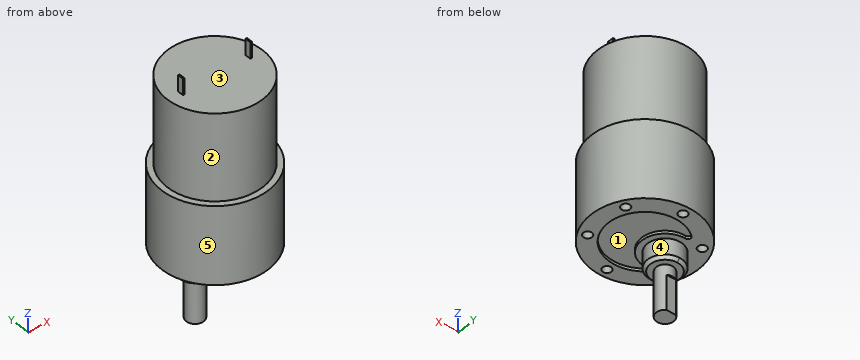
Autodesk Inventor part; units mm, degrees
ref_plane "YZ Plane" through (0, 0, 0) normal (1, 0, 0) x (0, 1, 0)
ref_plane "XZ Plane" through (0, 0, 0) normal (0, 1, 0) x (-1, 0, 0)
ref_plane "XY Plane" through (0, 0, 0) normal (0, 0, 1) x (1, 0, 0)
sketch "Boceto1" plane through (0, 0, 0) normal (0, 0, 1) x (1, 0, 0)
  circle A0 centre (0, 0) radius 18.4
  dimension "d0" = 36.8
extrude "Extrusión1" add sketch "Boceto1" along normal blind 27
sketch "Boceto2" plane through (0, 0, 27) normal (0, 0, 1) x (1, 0, 0)
  circle A0 centre (0, 0) radius 18.4
  circle A1 centre (0, 0) radius 16.4
  dimension "d4" = 2
extrude "Extrusión2" add sketch "Boceto2" along normal blind 30 contours A1
sketch "Boceto3" plane through (0, 0, 57) normal (0, 0, 1) x (1, 0, 0)
  circle A0 centre (0, 0) radius 16.4
  line L0 (0, 0) -> (12.05, 0)
  line L1 (0, 0) -> (-12.05, 0)
  line L2 (-12.05, 0) -> (-12.05, 1)
  line L3 (-12.05, 1) -> (-12, 1)
  line L4 (-12, 1) -> (-12, -1)
  line L5 (-12, -1) -> (-12.05, -1)
  line L6 (-12.05, -1) -> (-12.05, 0)
  line L7 (12.05, 0) -> (12.05, 1)
  line L8 (12.05, 1) -> (12, 1)
  line L9 (12, 1) -> (12, -1)
  line L10 (12, -1) -> (12.05, -1)
  line L11 (12.05, -1) -> (12.05, 0)
  dimension "d7" = 12.05
  dimension "d8" = 12.05
extrude "Extrusión3" add sketch "Boceto3" along normal blind 5.6 contours L9 L8 L7 L0 | L0 L11 L10 L9 | L4 L5 L6 L1 | L1 L2 L3 L4
sketch "Boceto4" plane through (0, 0, 0) normal (0, 0, -1) x (-1, 0, 0)
  circle A0 centre (13.4234, -7.75) radius 1.5
  circle A1 centre (13.4234, 7.75) radius 1.5
  circle A2 centre (0, 15.5) radius 1.5
  circle A3 centre (-13.4234, 7.75) radius 1.5
  circle A4 centre (-13.4234, -7.75) radius 1.5
  circle A5 centre (0, -15.5) radius 1.5
  line L0 (0, 0) -> (7, 0)
  circle A6 centre (7, 0) radius 6
  arc A7 (7.2895, 7.9948) -> (7.2895, -7.9948) centre (7, 0) ccw
  arc A8 (7.9572, 9.7695) -> (7.9572, -9.7695) centre (0, 0) ccw
  arc A9 (7.9572, -9.7695) -> (7.2895, -7.9948) centre (7.3257, -8.9941) ccw
  arc A10 (7.2895, 7.9948) -> (7.9572, 9.7695) centre (7.3257, 8.9941) ccw
  dimension "d19" = 7
  dimension "d20" = 12
  dimension "d34" = 1
extrude "Extrusión4" add sketch "Boceto4" along normal blind 6 contours A6
sketch "Boceto5" plane through (-7, 0, -6) normal (0, 0, -1) x (-1, 0, 0)
  circle A0 centre (0, 0) radius 6
  line L0 (6, 0) -> (0, 0)
  line L1 (0, 6) -> (0, 0)
extrude "Extrusión5" add sketch "Boceto5" along normal blind 0.5 contours L0 L1 A0 picked at (3.9499, 0.445)
sketch "Boceto6" plane through (0, 0, -6) normal (0, 0, -1) x (-1, 0, 0)
  line L0 (13, 0) -> (7, 0)
  line L1 (7, 0) -> (7, 6)
  arc A0 (7, 6) -> (13, 0) centre (7, 0) ccw
extrude "Extrusión6" cut sketch "Boceto6" against normal blind 0.5
sketch "Boceto7" plane through (-7, 0, -6.5) normal (1, 0, 0) x (0, 0, -1)
  line L0 (0, 0) -> (0, 6)
  line L1 (-1, 0) -> (0, 0)
  line L2 (-1, 6) -> (0, 5)
  line L3 (0, 5) -> (0, 6)
  line L4 (-1, 6) -> (0, 5)
  line L5 (-1, 6) -> (0, 6)
  line L6 (-1, 6) -> (0, 5)
  line L7 (0, 5) -> (-1, 6)
revolve "Revolución1" cut sketch "Boceto7" angle 360 about axis through (-7, 0, -5.5) along (0, 0, -1)
sketch "Boceto8" plane through (-7, 0, -5.5) normal (1, 0, 0) x (0, 0, -1)
  line L0 (1, 5) -> (0, 6)
  line L1 (0, 0) -> (0, 6)
  line L2 (0, 0) -> (1, 0)
  line L3 (1, 0) -> (1, 5)
revolve "Revolución2" add sketch "Boceto8" angle 360 about axis through (-7, 0, -5.5) along (0, 0, -1)
sketch "Boceto9" plane through (-7, 0, -6.5) normal (0, 0, -1) x (-1, 0, 0)
  circle A0 centre (0, 0) radius 5
  circle A1 centre (0, 0) radius 3
extrude "Extrusión7" add sketch "Boceto9" along normal blind 15.5 contours A1
sketch "Boceto10" plane through (-7, 0, -22) normal (0, 0, -1) x (-1, 0, 0)
  circle A0 centre (0, 0) radius 3
  line L0 (1.6583, 2.5) -> (-1.6583, 2.5)
extrude "Extrusión8" cut sketch "Boceto10" against normal blind 12 contours L0 A0 picked at (-0.1169, 2.6598)
extrude "Extrusión9" cut sketch "Boceto4" against normal blind 1 contours A7 A9 A8 A10
extrude "Extrusión10" cut sketch "Boceto4" against normal blind 10 contours A0 | A1 | A2 | A3 | A4 | A5
sketch "Boceto12" plane through (-12, -1, 57) normal (1, 0, 0) x (0, 0, -1)
  line L0 (-5.6, 2) -> (-5.6, 0)
  line L1 (0, 0) -> (-5.6, 0)
  line L2 (0, 2) -> (0, 0)
  line L3 (0, 2) -> (-5.6, 2)
extrude "Extrusión11" add sketch "Boceto12" along normal blind 0.45
sketch "Boceto13" plane through (12, -1, 57) normal (-1, 0, 0) x (0, 0, 1)
  line L0 (5.6, 0) -> (5.6, 2)
  line L1 (0, 2) -> (5.6, 2)
  line L2 (0, 0) -> (0, 2)
  line L3 (0, 0) -> (5.6, 0)
extrude "Extrusión12" add sketch "Boceto13" along normal blind 0.45
sketch "Boceto14" plane through (0, 0, 0) normal (0, 0, -1) x (-1, 0, 0)
  circle A0 centre (0, -15.5) radius 1.5
  circle A1 centre (-13.4234, -7.75) radius 1.5
  circle A2 centre (-13.4234, 7.75) radius 1.5
  circle A3 centre (13.4234, 7.75) radius 1.5
  circle A4 centre (13.4234, -7.75) radius 1.5
  circle A5 centre (0, 15.5) radius 1.5
  arc A6 (7.2895, 7.9948) -> (7.2895, -7.9948) centre (7, 0) ccw
  arc A7 (7.9572, -9.7695) -> (7.2895, -7.9948) centre (7.3257, -8.9941) ccw
  arc A8 (7.9572, 9.7695) -> (7.9572, -9.7695) centre (0, 0) ccw
  arc A9 (7.2895, 7.9948) -> (7.9572, 9.7695) centre (7.3257, 8.9941) ccw
  circle A10 centre (7, 0) radius 6
  circle A11 centre (0, 0) radius 18.4
sketch "Boceto15" plane through (-7, 0, -22) normal (0, 0, -1) x (-1, 0, 0)
  line L0 (1.6583, 2.5) -> (-1.6583, 2.5)
  arc A0 (-1.6583, 2.5) -> (1.6583, 2.5) centre (0, 0) ccw
properties part number "37D"
Work out the finished part from the listing and answer in its coordinate system (mm). Face numbers are marked on the shaded views. A direction names the side the tool comes from. Round coordinates to 2 decimals unless told otherwise and drop trailing zeros. Loops run counter-clockwise (first coordinate to the right, second up) from the corner with the lowest first, then second, coordinate; pieces in that order, holes last. Notation, with made-up numbers: M 62,69 L 104,69 A23 cw 104,84 Z; hole C 75.5,39 d1. An arc over 180 degrees is marked long. One line per question, with ' | ' between items.
Q1. Find section C-C, the plane z = 31. Give the vertices of the cut face in (x, y), then the cut area to 3 significant figures.
Conclusion:
outline: C 0,0 d32.8 | area: 845 mm2
Q2. Find section D-D, the plane y = -15.5. Give the vertices of the cut face in (x, z).
Conclusion:
outline: M -9.92,0 L -1.5,0 L -1.5,10 L 1.5,10 L 1.5,0 L 9.92,0 L 9.92,27 L 5.36,27 L 5.36,57 L -5.36,57 L -5.36,27 L -9.92,27 Z
Q3. Find section A-A, the plane y = 11. Give the vertices of the cut face in (x, z).
Conclusion:
outline: M -14.75,0 L -6.14,0 L -6.14,1 L 6.14,1 L 6.14,0 L 14.75,0 L 14.75,27 L 12.16,27 L 12.16,57 L -12.16,57 L -12.16,27 L -14.75,27 Z
Q4. Consider line 1 along Y through (x, z) = (0, 7.5); line 2 along Z through (x, y) = (16, 4.5); line 3 along Z through (x, y) = (-0.5, -6). Determine where each line is inside the solid, lowest interval first. Write a range as from..to.
Conclusion:
line 1: y = -18.4..-17, -14..14, 17..18.4 | line 2: z = 0..27 | line 3: z = 1..57
Q5. The mould has two halves that part along Y. Classify the marked faces 1, 2 and 3: +Y half, -Y half, draft (parallel to the pull), parting line (faces both ways), or undercut.
Conclusion:
face 1: undercut | face 2: parting line | face 3: draft
Q6. Find section B-B, the plane x = 0. Give the vertices of the cut face in (y, z).
Conclusion:
outline: M -18.4,0 L -17,0 L -17,10 L -14,10 L -14,0 L -12.6,0 L -12.6,1 L -3.87,1 L -3.87,0 L 3.87,0 L 3.87,1 L 12.6,1 L 12.6,0 L 14,0 L 14,10 L 17,10 L 17,0 L 18.4,0 L 18.4,27 L 16.4,27 L 16.4,57 L -16.4,57 L -16.4,27 L -18.4,27 Z
Q7. A tool of negligible diameter and unlimited length cuts with its end or side. For the marked faces 4 and 5, from which of +Z, -Z, +X, -X, +Y, -Y can it reach the whole face along a straight path? Write none if from no direction.
Conclusion:
face 4: -Z | face 5: +Z, -Z
Q8. Each of these flat-tipped pins is pushed along its axis until it touches: pin 1 Ø1 at (y, z) = (0, 60) entering from +X; pin 2 Ø0.6 at (x, y) = (-8, 3) entering from -Z; pin 3 Ø4 at (x, y) = (13.42, 7.75) entering from -Z. Where does it stop, or does it pass through?
Conclusion:
pin 1: stops at x = 12.05 | pin 2: stops at z = -10 | pin 3: stops at z = 0
